Input: part model. Units: mm. Frame: model coordinates. Coordinates: 2 decimals unless noted, no trailing zeros. Order: outer loops, then holes, each group sorted by start corner. A loop starts at its lowest first (then second) coordinate and runs counter-clockwise, first axis right, second up. Notation, with made-up numbers: (44.25, -9.5) - (77.25, -9.5) arc R23 cw to (77.25, 3.5) - close; hole circle Ø11 at (72, -11.75). An arc over 180 degrees is marked (long way). Use a Markdown table: item, result. Add a question column.
Autodesk Inventor part; units mm, degrees
ref_plane "YZ Plane" through (0, 0, 0) normal (1, 0, 0) x (0, 1, 0)
ref_plane "XZ Plane" through (0, 0, 0) normal (0, 1, 0) x (-1, 0, 0)
ref_plane "XY Plane" through (0, 0, 0) normal (0, 0, 1) x (1, 0, 0)
sketch "Эскиз1" plane through (0, 0, 0) normal (0, 0, 1) x (1, 0, 0)
  line L0 (52, 11) -> (0, 11)
  line L1 (0, -11) -> (52, -11)
  arc A0 (52, 11) -> (52, -11) centre (52, 0) ccw
  line L2 (0, -11) -> (0, 11)
  line L3 (0, 0) -> (41, 0) construction
  line L4 (0, 0) -> (0, 11) construction
  line L5 (0, 11) -> (0, 11.25)
  point P0 (20.5, 0)
  dimension "d0" = 11
  dimension "d47" = 41
extrude "Выдавливание3" add sketch "Эскиз1" along normal blind 1.4
fillet "Сопряжение3" radius 0.25 2 edges at (52, 11, 0.7) (52, -11, 0.7)
fillet "Сопряжение4" radius 3.5 2 edges at (0, -11, 0.7) (0, 11, 0.7)
sketch "Эскиз6" plane through (0, 0, 1.4) normal (0, 0, 1) x (1, 0, 0)
  arc A0 (48.7571, 10.5111) -> (48.7571, -10.5111) centre (52, 0) ccw construction
  line L0 (41, 0) -> (0, 0) construction
  line L1 (0, -11) -> (0, 11) construction
  circle A1 centre (3.5, 3.5) radius 0.5
  line L2 (3.5, 3.5) -> (0, 3.5) construction
  line L3 (3.5, 3.5) -> (3.5, 0) construction
  circle A2 centre (3.5, -3.5) radius 0.5
  point P0 (48.6834, -11)
  dimension "d58" = 1
  dimension "d59" = 3.5
hole "Отверстие1" at (3.5, -3.5, 1.4) at (3.5, 3.5, 1.4) direction (0, 0, -1) diameter 1 end through all countersink diameter 1.5 countersink angle 90
properties part number "Поршень"
1) Cut plane A-A (z = 0.7). Return the cut outline in (x, y), and give its area (3 significant figures).
2) Cut plane B-B (y = -3.5). Return the cut outline in (x, z), and give its area (3 significant figures).
3) Pull-direction query (Y, two-part tool) for faces 1 (the flat face through (24, 0, 0)), 2 (the flat face through (26, -11, 1)), 3 (the flat face through (26, 11, 1)), 4 (the cylindrical face through (3.2, -3.1, 0.6)); classes: pulls with the +Y half, pulls with the -Y half, needs draft (parallel to the pull), parting line crosses it, or undercut.
4) Material intervals for L1, parallel to Y at x = 3.5, z = 0.4; L2, parallel to X at y = 3.5, z = 0.85; L3, parallel to Y at x = 46.5, z = 0.15, sorted ascending.
5) Contact query for a flat-ended pin moving along its axis: P1, Ø4, axis at x = 14, y = 0.5, coming from the -Z side. Output: stop coordinate, or through.
Computed:
| question | item | result |
|---|---|---|
| 1 | outline | (0, -7.5) arc R3.5 ccw to (3.5, -11) - (48.68, -11) arc R0.25 ccw to (48.76, -10.51) arc R11 cw to (48.76, 10.51) arc R0.25 ccw to (48.68, 11) - (3.5, 11) arc R3.5 ccw to (0, 7.5) - close; hole circle Ø1 at (3.5, -3.5); hole circle Ø1 at (3.5, 3.5) |
| 1 | area | 946 mm2 |
| 2 | outline | (0, 0) - (3, 0) - (3, 1.15) - (2.75, 1.4) - (0, 1.4) - close; (4, 0) - (41.57, 0) - (41.57, 1.4) - (4.25, 1.4) - (4, 1.15) - close |
| 2 | area | 56.7 mm2 |
| 3 | face 1 | needs draft |
| 3 | face 2 | pulls with the -Y half |
| 3 | face 3 | pulls with the +Y half |
| 3 | face 4 | undercut |
| 4 | L1 | y = -11 to -4, -3 to 3, 4 to 11 |
| 4 | L2 | x = 0 to 3, 4 to 41.57 |
| 4 | L3 | y = -11 to -9.53, 9.53 to 11 |
| 5 | P1 | stops at z = 0 |
